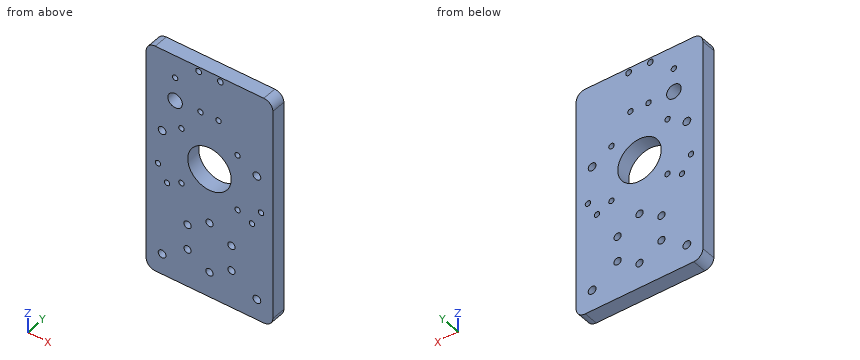
Autodesk Inventor part; units mm, degrees
ref_plane "YZ Plane" through (0, 0, 0) normal (1, 0, 0) x (0, 1, 0)
ref_plane "XZ Plane" through (0, 0, 0) normal (0, 1, 0) x (-1, 0, 0)
ref_plane "XY Plane" through (0, 0, 0) normal (0, 0, 1) x (1, 0, 0)
sketch "Sketch1" plane through (0, 0, 0) normal (0, 1, 0) x (-1, 0, 0)
  line L0 (35, 99.5) -> (-35, 99.5)
  line L1 (-35, 99.5) -> (-35, -27.999)
  line L2 (-35, -27.999) -> (35, -27.999)
  line L3 (35, -27.999) -> (35, 99.5)
  line L4 (26.1865, 53.5) -> (-26.1865, 53.5) construction
  line L5 (-26.1865, 53.5) -> (-26.1865, -16.5) construction
  line L6 (-26.1865, -16.5) -> (26.1865, -16.5) construction
  line L7 (26.1865, -16.5) -> (26.1865, 53.5) construction
  circle A0 centre (26.1865, 53.5) radius 4 construction
  circle A1 centre (-26.1865, 53.5) radius 4 construction
  circle A2 centre (-26.1865, -16.5) radius 4 construction
  circle A3 centre (26.1865, -16.5) radius 4 construction
  circle A4 centre (0, 40) radius 15 construction
  line L8 (20.5, 20.5) -> (-20.5, 20.5) construction
  line L9 (-20.5, 20.5) -> (-20.5, -20.5) construction
  line L10 (-20.5, -20.5) -> (20.5, -20.5) construction
  line L11 (20.5, -20.5) -> (20.5, 20.5) construction
  point P0 (0, 0)
  dimension "d57" = 127.499
  dimension "d58" = 70
  dimension "d59" = 8
  dimension "d60" = 8
  dimension "d61" = 8
  dimension "d62" = 8
  dimension "d63" = 70
  dimension "d64" = 52.373
  dimension "d66" = 8.8135
  dimension "d67" = 46
  dimension "d70" = 30
  dimension "d71" = 41
  dimension "d72" = 41
  dimension "d73" = 20.5
  dimension "d74" = 20.5
  dimension "d75" = 40
  dimension "d76" = 35
  dimension "d210" = 16.5
extrude "Extrusion1" add sketch "Sketch1" along normal blind 8
sketch "Sketch7" plane through (0, 8, 0) normal (0, 1, 0) x (1, 0, 0)
  circle A0 centre (0, -44.501) radius 12
  line L0 (35, 27.999) -> (-35, 27.999)
  line L1 (-35, 27.999) -> (-35, -99.5)
  dimension "d77" = 24
  dimension "d205" = 72.5
  dimension "d206" = 35
hole "MotormainHole5" at (0, 8, 44.501) direction (0, -1, 0) diameter 24 end through all
sketch "Sketch8" plane through (0, 8, 0) normal (0, 1, 0) x (1, 0, 0)
  line L0 (15.5, -60.001) -> (-15.5, -60.001) construction
  line L1 (-15.5, -60.001) -> (-15.5, -29.001) construction
  line L2 (-15.5, -29.001) -> (15.5, -29.001) construction
  line L3 (15.5, -29.001) -> (15.5, -60.001) construction
  circle A0 centre (15.5, -60.001) radius 1.5
  circle A1 centre (-15.5, -60.001) radius 1.5
  circle A2 centre (-15.5, -29.001) radius 1.5
  circle A3 centre (15.5, -29.001) radius 1.5
  circle A4 centre (0, -44.501) radius 12
  point P0 (0, 0)
  dimension "d85" = 3
  dimension "d86" = 31
  dimension "d87" = 31
  dimension "d88" = 15.5
  dimension "d215" = 15.5
hole "MotorHole6" at (15.5, 8, 60.001) at (-15.5, 8, 60.001) at (-15.5, 8, 29.001) at (15.5, 8, 29.001) direction (0, -1, 0) diameter 3 end through all
sketch "Sketch9" plane through (0, 0, 0) normal (0, -1, 0) x (1, 0, 0)
  circle A0 centre (-5, 74.501) radius 1.5
  circle A1 centre (5, 74.501) radius 1.5
  line L0 (-35, -27.999) -> (-35, 99.5)
  line L1 (35, 99.5) -> (35, -27.999)
  circle A2 centre (0, 44.501) radius 12
  point P0 (0, 0)
  dimension "d97" = 3
  dimension "d186" = 30
  dimension "d187" = 30
  dimension "d207" = 30
hole "GrippersupportHole7" at (-5, 0, 74.501) at (5, 0, 74.501) direction (0, 1, 0) diameter 3 end through all
sketch "Sketch10" plane through (0, 8, 0) normal (0, 1, 0) x (1, 0, 0)
  line L0 (26.1865, -53.5) -> (-26.1865, -53.5) construction
  line L1 (-26.1865, -53.5) -> (-26.1865, 16.5) construction
  line L2 (-26.1865, 16.5) -> (26.1865, 16.5) construction
  line L3 (26.1865, 16.5) -> (26.1865, -53.5) construction
  circle A0 centre (26.1865, -53.5) radius 2.15
  circle A1 centre (-26.1865, -53.5) radius 2.15
  circle A2 centre (-26.1865, 16.5) radius 2.15
  circle A3 centre (26.1865, 16.5) radius 2.15
  line L4 (35, -99.5) -> (35, 27.999)
  line L5 (-35, -99.5) -> (35, -99.5)
  point P0 (0, 0)
  dimension "d111" = 4.3
  dimension "d112" = 8.8135
  dimension "d113" = 52.373
  dimension "d114" = 46
  dimension "d115" = 70
hole "supportHole8" at (26.1865, 8, 53.5) at (-26.1865, 8, 53.5) at (26.1865, 8, -16.5) at (-26.1865, 8, -16.5) direction (0, -1, 0) diameter 4.3 end through all
sketch "Sketch11" plane through (0, 0, 0) normal (0, -1, 0) x (1, 0, 0)
  circle A0 centre (0, 0) radius 14 construction
  circle A1 centre (-26.1865, 53.5) radius 2.15
  circle A2 centre (26.1865, 53.5) radius 2.15
  circle A3 centre (0, 14) radius 2
  circle A4 centre (-12.1244, 7) radius 2
  circle A5 centre (-12.1244, -7) radius 2
  circle A6 centre (0, -14) radius 2
  line L0 (35, -27.999) -> (-35, -27.999)
  circle A7 centre (-26.1865, -16.5) radius 2.15
  circle A8 centre (26.1865, -16.5) radius 2.15
  circle A9 centre (12.1244, -7) radius 2
  circle A10 centre (12.1244, 7) radius 2
  point P0 (0, 0)
  dimension "d125" = 28
  dimension "d126" = 4
  dimension "d129" = 360
  dimension "d213" = 16.5
  dimension "d214" = 0
hole "ScrewHole9" at (0, 0, 14) at (0, 0, -14) at (-12.1244, 0, -7) at (-12.1244, 0, 7) direction (0, 1, 0) diameter 4 end through all
fillet "MainFillet1" radius 5 4 edges at (-35, 4, 99.5) (35, 4, 99.5) (35, 4, -27.999) (-35, 4, -27.999)
sketch "Sketch12" plane through (0, 8, 0) normal (0, 1, 0) x (1, 0, 0)
  circle A0 centre (-19, -74) radius 4
  point P0 (0, 0)
  dimension "d139" = 8
  dimension "d140" = 19
  dimension "d141" = 74
hole "Wirehole" at (-19, 8, 74) direction (0, -1, 0) diameter 8 end through all
sketch "Sketch13" plane through (0, 0, 0) normal (0, -1, 0) x (1, 0, 0)
  circle A0 centre (-19, 87) radius 1.5
  circle A1 centre (-19, 74) radius 4
  line L0 (-19, 74) -> (-19, 90.0353) construction
  line L1 (-19, 74) -> (-19, 87) construction
  point P0 (0, 0)
  dimension "d149" = 3
  dimension "d211" = 13
  dimension "d212" = 0
hole "Hole11" at (-19, 0, 87) direction (0, 1, 0) diameter 3 end through all
sketch "Sketch16" plane through (0, 8, 0) normal (0, 1, 0) x (1, 0, 0)
  circle A0 centre (-6, -97) radius 1.6
  circle A1 centre (6, -97) radius 1.6
  line L0 (-30, -99.5) -> (30, -99.5)
  circle A2 centre (-26.1865, -53.5) radius 2.15
  point P0 (0, 0)
  point P1 (-20, -99.5)
  dimension "d173" = 3.2
  dimension "d174" = 12
  dimension "d175" = 6
  dimension "d216" = 43.5
hole "chainHole13" at (-6, 8, 97) at (6, 8, 97) direction (0, -1, 0) diameter 3.2 end through all
sketch "Sketch17" plane through (0, 8, 0) normal (0, 1, 0) x (1, 0, 0)
  circle A0 centre (-5, -74.501) radius 1.5
  circle A1 centre (5, -74.501) radius 1.5
  circle A2 centre (-5, -74.501) radius 1.5
  circle A3 centre (5, -74.501) radius 1.5
  circle A4 centre (28.4808, -33.8311) radius 1.5
  circle A5 centre (23.4808, -25.1709) radius 1.5
  circle A6 centre (-23.4808, -25.1709) radius 1.5
  circle A7 centre (-28.4808, -33.8311) radius 1.5
  circle A8 centre (0, -44.501) radius 12
  dimension "d188" = 0
  dimension "d189" = 0
  dimension "d190" = 3
  dimension "d193" = 360
  dimension "d208" = 0
  dimension "d209" = 0
hole "Grippersupport2Hole14" at (23.4808, 8, 25.1709) at (28.4808, 8, 33.8311) at (-28.4808, 8, 33.8311) at (-23.4808, 8, 25.1709) direction (0, -1, 0) diameter 3 end through all
sketch "Sketch18" plane through (0, 8, 0) normal (0, 1, 0) x (1, 0, 0)
  circle A0 centre (0, 0) radius 14
  line L0 (0, 0) -> (16.8596, -9.7339)
  line L1 (0, 0) -> (20.1281, 11.6209)
  line L2 (0, 0) -> (0, -20)
  point P0 (12.1244, 7)
  point P1 (12.1244, -7)
  dimension "d217" = 28
  dimension "d218" = 20
  dimension "d219" = 60
  dimension "d220" = 120
hole "Hole15" at (12.1244, 8, 7) at (12.1244, 8, -7) direction (0, -1, 0) diameter 4 end through all
equation "\"d66\" = -0.5 * d64 + 0.5 * d58"
equation "\"d78\" = d77"
equation "\"d90\" = d85"
equation "\"d101\" = d97"
equation "\"d112\" = d66"
equation "\"d113\" = d64"
equation "\"d114\" = d67"
equation "\"d115\" = d63"
equation "\"d116\" = d111"
equation "\"d142\" = d139"
equation "\"d177\" = d173"
equation "\"d195\" = d190"
properties part number "Gripper_Base_new" material "PET Plastic"
Check sheet for the modelled part. Datum: model origin and axes. Units: mm. Round coordinates to 2 decimals unless told otherwise and drop trailing zeros. Order: outer loops, then holes, each group sorted by start corner. A loop starts at its lowest first (then second) coordinate and runs counter-clockwise, first axis right, second up. Notation, with made-up numbers: (-29, 75) -> (0, 75) arc R15 cw to (0, 101) -> close; hole circle Ø4 at (22, -11.75). An arc over 180 degrees is marked (long way). One line per item, written item: value. Start each with the question number.
Q1. Cross-section at C-C (x = 15.5). Record the boundary of the cut face in (y, z), and give its area (3 significant figures).
Q2. Gauge pin test, flat end, axial feed: pin 1 Ø1.8 at (x, z) = (-28.48, 33.83) entering from +Y. Record the tip position at first contact, or that the pin passes through.
Q3. Thickness scan on line 1 (Z direction, x = 0, y = 3.5); line 2 (X direction, y = 2.25, z = 45); line 3 (Z direction, x = -5, y = 7.5). Record the ranges inside material, lowest first.
Q4. Cross-section at A-A (z = -7). Record the boundary of the cut face in (x, y).
Q5. Cross-section at D-D (z = 53.5). Record the boundary of the cut face in (x, y).
Q6. Cross-section at B-B (z = 87). Record the boundary of the cut face in (x, y), and give its area (3 significant figures).
Completed:
1. outline: (0, -28) -> (8, -28) -> (8, 27.5) -> (0, 27.5) -> close; (0, 30.5) -> (8, 30.5) -> (8, 58.5) -> (0, 58.5) -> close; (0, 61.5) -> (8, 61.5) -> (8, 99.5) -> (0, 99.5) -> close
1. area: 972 mm²
2. pin 1: passes through
3. line 1: z = -28 to -16, -12 to 12, 16 to 32.5, 56.5 to 99.5
3. line 2: x = -35 to -11.99, 11.99 to 35
3. line 3: z = -28 to 33.59, 55.41 to 73, 76 to 95.75, 98.25 to 99.5
4. outline: (-35, 0) -> (-14.12, 0) -> (-14.12, 8) -> (-35, 8) -> close; (-10.12, 0) -> (10.12, 0) -> (10.12, 8) -> (-10.12, 8) -> close; (14.12, 0) -> (35, 0) -> (35, 8) -> (14.12, 8) -> close
5. outline: (-35, 0) -> (-28.34, 0) -> (-28.34, 8) -> (-35, 8) -> close; (-24.04, 0) -> (-7.94, 0) -> (-7.94, 8) -> (-24.04, 8) -> close; (7.94, 0) -> (24.04, 0) -> (24.04, 8) -> (7.94, 8) -> close; (28.34, 0) -> (35, 0) -> (35, 8) -> (28.34, 8) -> close
6. outline: (-35, 0) -> (-20.5, 0) -> (-20.5, 8) -> (-35, 8) -> close; (-17.5, 0) -> (35, 0) -> (35, 8) -> (-17.5, 8) -> close
6. area: 536 mm²
